Study the drawing (mm; zero at the part's minimum x, y, z) and answer. Coordinates: 2 decimals unless noted, no trailing zeros. Loops run counter-clockwise (first coordinate to the right, second up) from the corner with the lowest first, then second, coordinate; pieces in that order, holes last. Notation, with made-up numbers: (48, -14) - (101, -14) arc R23 cw to (101, 1) - close; hole circle Ø4 at (32.25, -11.75). An arc over 180 degrees is marked (long way). Use one line per item in the form item = value.
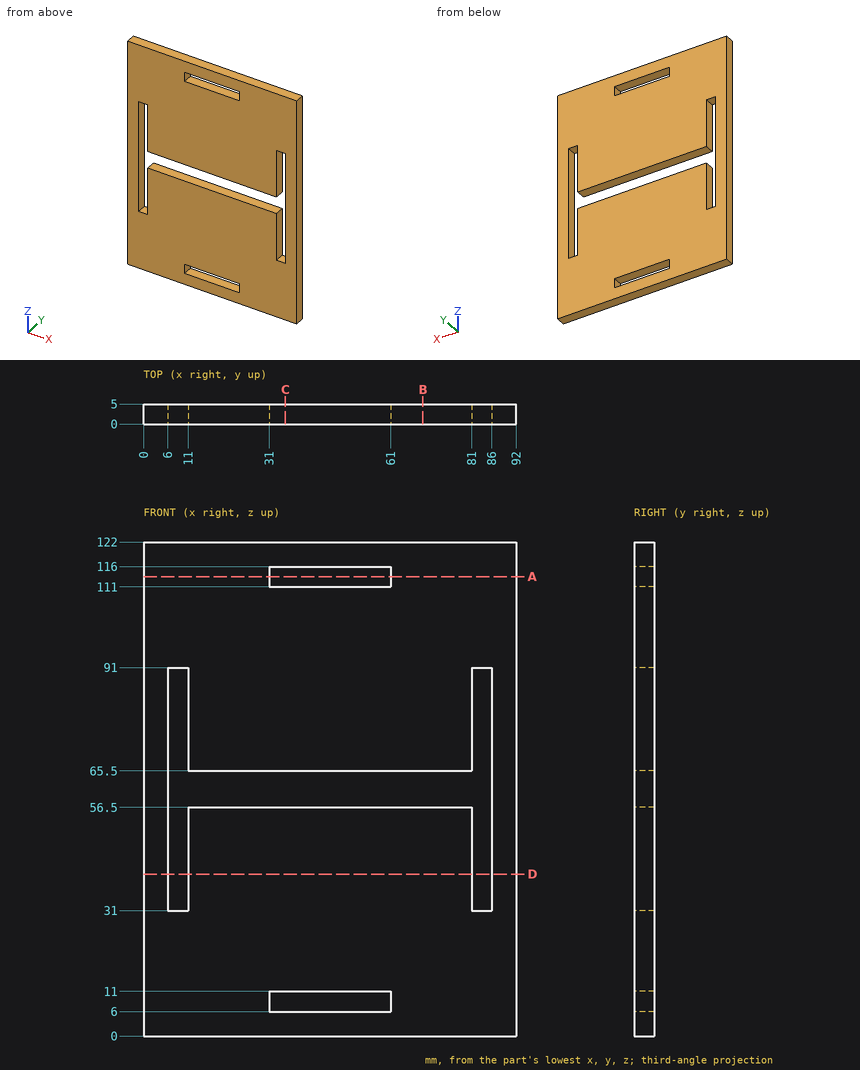
Item 1: Find the intervals of material crossed by L1, parallel to X at y = 3.7, z = 34; L2, parallel to Z at x = 51, y = 3.4; L3, parallel to Z at x = 7, y = 3.35, in increasing order.
Results below:
L1 = 0 to 6, 11 to 81, 86 to 92
L2 = 0 to 6, 11 to 56.5, 65.5 to 111, 116 to 122
L3 = 0 to 31, 91 to 122
Item 2: The part is cut by section A-A on z = 113.5. Give the vertices of the cut face in (x, y), plus the area to 3 significant figures.
Results below:
outline = (0, 0) - (31, 0) - (31, 5) - (0, 5) - close; (61, 0) - (92, 0) - (92, 5) - (61, 5) - close
area = 310 mm²
Item 3: The part is cut by section B-B on x = 69. Give the vertices of the cut face in (y, z).
Results below:
outline = (0, 0) - (5, 0) - (5, 56.5) - (0, 56.5) - close; (0, 65.5) - (5, 65.5) - (5, 122) - (0, 122) - close
Item 4: The part is cut by section D-D on z = 40. Give the vertices of the cut face in (x, y), plus the area to 3 significant figures.
Results below:
outline = (0, 0) - (6, 0) - (6, 5) - (0, 5) - close; (11, 0) - (81, 0) - (81, 5) - (11, 5) - close; (86, 0) - (92, 0) - (92, 5) - (86, 5) - close
area = 410 mm²
Item 5: The part is cut by section C-C on x = 35. Give the vertices of the cut face in (y, z).
Results below:
outline = (0, 0) - (5, 0) - (5, 6) - (0, 6) - close; (0, 11) - (5, 11) - (5, 56.5) - (0, 56.5) - close; (0, 65.5) - (5, 65.5) - (5, 111) - (0, 111) - close; (0, 116) - (5, 116) - (5, 122) - (0, 122) - close
